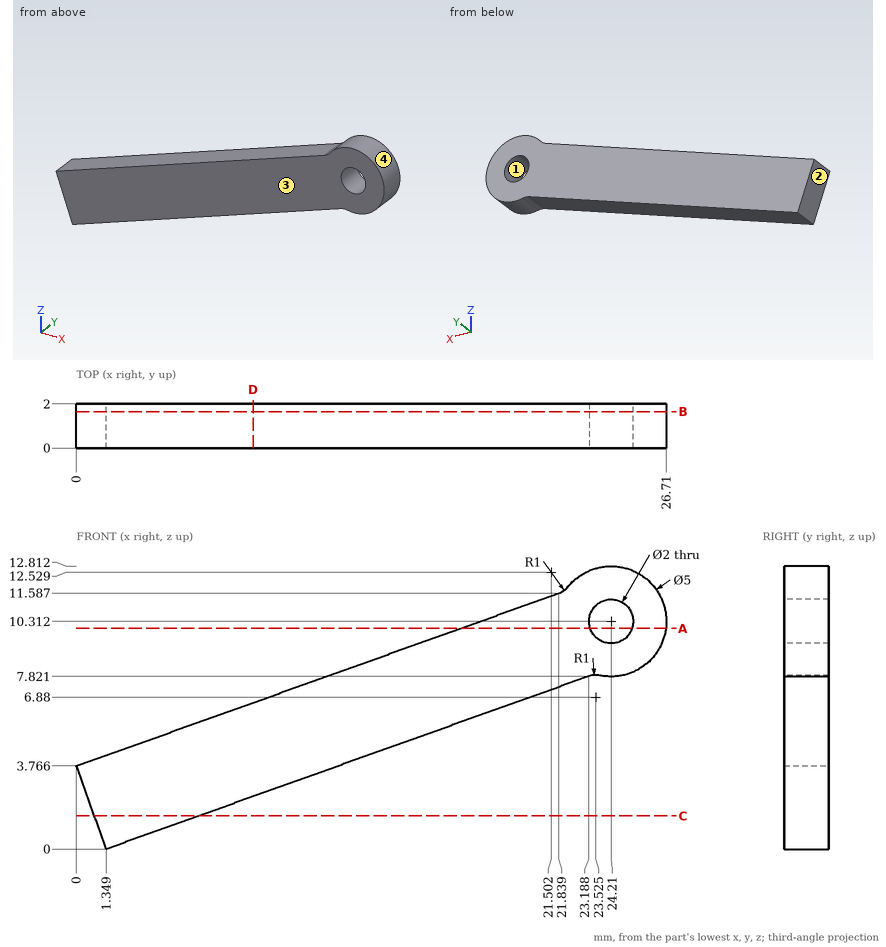
Could you check a few things on this drawing? It's one solid part, dimensions in mm from its lowest x, y, z. Give positions to 0.01 mm unless a question says otherwise; leave off trailing zeros. Order: outer loops, then holes, each group sorted by start corner. A loop starts at its lowest first (then second) coordinate and runs counter-clockwise, first axis right, second up. Notation, with made-up numbers: (73, -11.75) - (101, -11.75) arc R24 cw to (101, 8.25) - close; hole circle Ø3 at (-10.75, -31.75). An arc over 180 degrees is marked (long way). Return JSON: item names as keys, results as strings. Group by question number.
Q1. Suppose I cut it at D-D, the plane x = 8. Please give me the cut outline in (y, z).
Q2. Thinking about a two-plate mould opening in Z: for the marked faces 1, 2, 3 and 4, which applies, pulls with the +Z half, pulls with the -Z half, needs draft (parallel to the pull), parting line crosses it, or undercut?
Q3. Will this pin go through, and if not, where does the flat tip stop? pin 1 Ø1 at (x, y) = (11, 1) entering from -Z.
Q4. Suppose I cut it at B-B, the plane y = 1.65. Please give me the cut outline in (x, z) (1 decimal), and give its area (3 significant figures).
Q5. Please list where these lines run through material, in increasing order: line 1 along Z through (x, y) = (24.25, 0.55); line 2 along Z through (x, y) = (15.75, 1.1) (1 decimal); line 3 along Z through (x, y) = (18, 1.8) (1 decimal). Write a range as [from, to].
Q6. Suppose I cut it at A-A, the plane z = 10. Please give me the cut outline in (x, y).
Q7. Suppose I cut it at C-C, the plane z = 1.5. Please give me the cut outline in (x, y).
Resolved:
{
 "1": {"outline": "(0, 2.38) - (2, 2.38) - (2, 6.63) - (0, 6.63) - close"},
 "2": {"face 1": "undercut", "face 2": "pulls with the -Z half", "face 3": "needs draft", "face 4": "parting line crosses it"},
 "3": {"pin 1": "stops at z = 3.28"},
 "4": {"outline": "(0, 3.8) - (1.3, 0) - (23.2, 7.8) arc R1 cw to (23.7, 7.9) arc R2.5 ccw (long way) to (22.3, 11.9) arc R1 cw to (21.8, 11.6) - close; hole circle Ø2 at (24.2, 10.3)", "area": "108 mm2"},
 "5": {"line 1": "z = [7.81, 9.31], [11.31, 12.81]", "line 2": "z = [5.2, 9.4]", "line 3": "z = [6, 10.2]"},
 "6": {"outline": "(17.41, 0) - (23.26, 0) - (23.26, 2) - (17.41, 2) - close; (25.16, 0) - (26.69, 0) - (26.69, 2) - (25.16, 2) - close"},
 "7": {"outline": "(0.81, 0) - (5.54, 0) - (5.54, 2) - (0.81, 2) - close"}
}
